The model under review builds one solid part; all positions refer to its coordinate system, in mm. Face numbers are marked on the shaded views. A direction names the side the tool comes from. Coordinates: 2 decimals unless noted, no trailing zeros. Order: outer loops, then holes, each group sorted by start corner. A loop starts at its lowest first (then second) coordinate and runs counter-clockwise, first axis right, second up.
```python
from build123d import *

# Parameters (mm, degrees)
SKETCH_1_W          = 54
SKETCH_1_H          = 100
EXTRUDE_1_DEPTH     = 60
SKETCH_2_W          = 54
SKETCH_2_H          = 60
EXTRUDE_2_DEPTH     = 22.5
SKETCH_3_W          = 8.5
SKETCH_3_H          = 12.5
CUT_EXTRUDE_1_DEPTH = 22.5
CUT_EXTRUDE_2_DEPTH = 10
CUT_EXTRUDE_3_DEPTH = 10


with BuildPart() as part:
    # 草图1 → 凸台-拉伸1 (new body)
    with BuildSketch(Plane.XY):
        with Locations((-27, -50)):
            Rectangle(SKETCH_1_W, SKETCH_1_H)
    extrude(amount=EXTRUDE_1_DEPTH)

    # 草图2 → 凸台-拉伸2 (add)
    with BuildSketch(Plane.XY.offset(60)):
        with Locations((-27, -40)):
            Rectangle(SKETCH_2_W, SKETCH_2_H)
    extrude(amount=EXTRUDE_2_DEPTH)

    # 草图3 → 切除-拉伸1 (cut)
    with BuildSketch(Plane(origin=(0, -10, 0), x_dir=(1, 0, 0), z_dir=(0, 1, 0))):
        with Locations((-12.25, -69.25)):
            Rectangle(SKETCH_3_W, SKETCH_3_H)
    extrude(amount=-CUT_EXTRUDE_1_DEPTH, mode=Mode.SUBTRACT)

    # 草图4 → 切除-拉伸2 (cut)
    with BuildSketch(Plane(origin=(0, 0, 0), x_dir=(1, 0, 0), z_dir=(0, 1, 0))):
        with BuildLine():
            Line((-37, -27), (-37, -47))
            ThreePointArc((-37, -47), (-39, -49), (-41, -47))
            Line((-41, -47), (-41, -27))
            ThreePointArc((-41, -27), (-39, -25), (-37, -27))
        make_face()
        with BuildLine():
            Line((-17, -27), (-17, -47))
            ThreePointArc((-17, -47), (-15, -49), (-13, -47))
            Line((-13, -47), (-13, -27))
            ThreePointArc((-13, -27), (-15, -25), (-17, -27))
        make_face()
    extrude(amount=-CUT_EXTRUDE_2_DEPTH, mode=Mode.SUBTRACT)

    # 草图5 → 切除-拉伸3 (cut)
    with BuildSketch(Plane(origin=(0, 0, 0), x_dir=(0, 0, -1), z_dir=(1, 0, 0))):
        Polygon((-44.403805922, -8), (-19.5, -8), (-19.5, -32.903805922), align=None)
        Polygon((-24.096194078, -37.5), (-49, -12.596194078), (-49, -37.5), align=None)
    extrude(amount=-CUT_EXTRUDE_3_DEPTH, mode=Mode.SUBTRACT)


solid = part.part
```
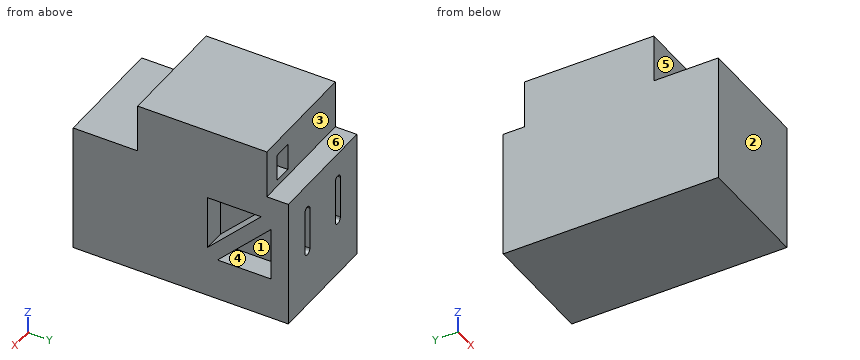
(1) Wall thickness on probe 1 along Z at (x, y) = (-39, -4.5); probe 2 along Y at (x, z) = (-5, 37.5); probe 3 along Y at (x, z) = (-34, 69): over which ranges is each line inside the solid? List them lowest first.
A:
probe 1: z = 0 to 25, 49 to 60
probe 2: y = -100 to -37.5, -24.1 to -14.9, -8 to 0
probe 3: y = -70 to -10
(2) We need section C-C, the plane z = 35. Write out the cut boundary in (x, y).
A:
outline: (-54, -100) - (0, -100) - (0, -37.5) - (-10, -37.5) - (-10, -26.6) - (0, -26.6) - (0, -17.4) - (-10, -17.4) - (-10, -8) - (0, -8) - (0, 0) - (-13, 0) - (-13, -10) - (-17, -10) - (-17, 0) - (-37, 0) - (-37, -10) - (-41, -10) - (-41, 0) - (-54, 0) - close
(3) Machinability: for the marked faces 4, 5 and 6, which of the approach directions +Z, -Z, +X, -X, +Y, -Y give a long, thin tool a straight path to every point of the face, cutting with its end or side? Answer none if there is none.
A:
face 4: +X
face 5: +Z, +X, -X, -Y
face 6: +Z, +X, -X, +Y
(4) Draft analysis for pull direction Y (two halves, no side actions). For the marked faces 1, 2 and 3, state which applies: released by +Y, released by -Y, zero draft, split by the parting line, or undercut.
A:
face 1: undercut
face 2: released by -Y
face 3: released by +Y
(5) We need section D-D, the plane y = -71.5. Write out the cut boundary in (x, z).
A:
outline: (-54, 0) - (0, 0) - (0, 60) - (-54, 60) - close
(6) We need section A-A, the plane x = -15. Write out the cut boundary in (y, z), and give its area (3 significant figures).
A:
outline: (-100, 0) - (0, 0) - (0, 25) - (-10, 25) - (-10, 49) - (0, 49) - (0, 60) - (-10, 60) - (-10, 63) - (-32.5, 63) - (-32.5, 75.5) - (-10, 75.5) - (-10, 82.5) - (-70, 82.5) - (-70, 60) - (-100, 60) - close
area: 6,830 mm2
(7) We need section B-B, the plane x = -39. Write out the cut boundary in (y, z), and give its area (3 significant figures).
A:
outline: (-100, 0) - (0, 0) - (0, 25) - (-10, 25) - (-10, 49) - (0, 49) - (0, 60) - (-10, 60) - (-10, 82.5) - (-70, 82.5) - (-70, 60) - (-100, 60) - close
area: 7,110 mm2
(8) For pin 1 Ø3 at (x, z) = (-39, 33.5) entering from +Y; pin 2 Ø18 at (x, z) = (-37, 72) entering from -Y; pin 3 Ø4 at (x, z) = (-11, 68.5) entering from +Y, all flat-tipped, find the tip position at first contact; note any pin that passes through.
A:
pin 1: stops at y = -10
pin 2: stops at y = -70
pin 3: stops at y = -32.5
